Check sheet for the drawn part. Datum: minimum x, y, z corner. Units: mm. Coordinates: 2 decimals unless noted, no trailing zeros. Order: outer loops, then holes, each group sorted by start corner. A loop starts at its lowest first (then second) coordinate and runs counter-clockwise, first axis right, second up. Notation, with made-up numbers: M 0,69 L 30,69 A19 ccw 30,92 Z; hole C 60,59.5 d9. An arc over 180 degrees is marked long. Return JSON: item names as keys, results as strings. Group by question number.
Q1. Thickness scan on probe 1 along X at (y, z) = (6.5, 1.6); probe 2 along Y at (x, z) = (26, 0.4); probe 3 along X at (y, z) = (41, 3.6). Record the ranges inside material, lowest first.
Q2. Section check A-A, the plane y = 15. Enter the section's corners in (x, z).
Q3. Go/stop test with flat-tipped pins: pin 1 Ø1.1 at (x, z) = (6, 2.5) entering from -Y; pin 2 Ø2 at (x, z) = (75.5, 2.5) entering from -Y. Record where each tip stops, or that it passes through.
Q4. Section check C-C, the plane x = 69. Enter the section's corners in (y, z).
Q5. Section check B-B, the plane z = 1.7. Enter the section's corners in (x, y).
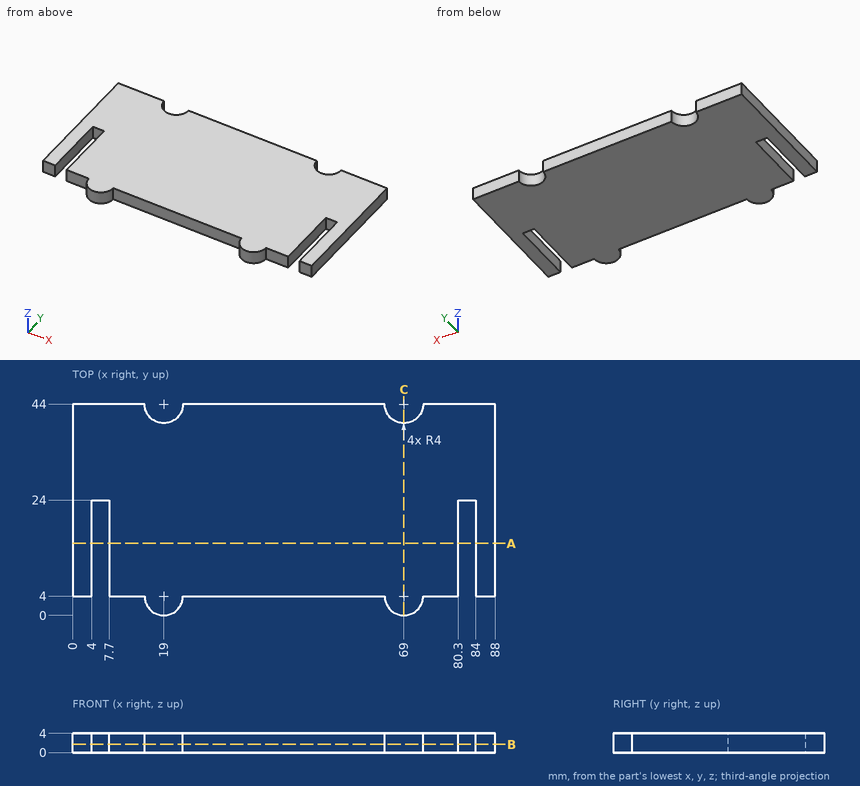
Numbers:
{
 "1": {"probe 1": "x = 0 to 4, 7.7 to 80.3, 84 to 88", "probe 2": "y = 4 to 44", "probe 3": "x = 0 to 16.35, 21.65 to 66.35, 71.65 to 88"},
 "2": {"outline": "M 0,0 L 4,0 L 4,4 L 0,4 Z; M 7.7,0 L 80.3,0 L 80.3,4 L 7.7,4 Z; M 84,0 L 88,0 L 88,4 L 84,4 Z"},
 "3": {"pin 1": "stops at y = 24", "pin 2": "stops at y = 4"},
 "4": {"outline": "M 0,0 L 40,0 L 40,4 L 0,4 Z"},
 "5": {"outline": "M 0,4 L 4,4 L 4,24 L 7.7,24 L 7.7,4 L 15,4 A4 ccw 23,4 L 65,4 A4 ccw 73,4 L 80.3,4 L 80.3,24 L 84,24 L 84,4 L 88,4 L 88,44 L 73,44 A4 cw 65,44 L 23,44 A4 cw 15,44 L 0,44 Z"}
}
